Design review of the part built by this model. Coordinates are the model's own, in mm. Give positions to 0.01 mm unless a question says otherwise; leave off trailing zeros. Write each loop counter-clockwise with the first axis right and the second up, starting at its lowest first coordinate (ties: lowest second). Pieces come first, ordered by that corner, then holes. Notation, with made-up numbers: M 65.5,35.25 L 116.5,35.25 A15 cw 116.5,48.25 Z; hole C -4.5,1 d2. An arc over 180 degrees is marked long. Write each question's results on one line, items separated by ' | '. Start each with the question number.
from build123d import *

# Parameters (mm, degrees)
F0_W     = 15
F0_H     = 3.175
F0_W_2   = 10
F0_W_3   = 11
F0_H_2   = 20
F1_DEPTH = 3.175
F2_R     = 5


# Not quite as in the source:
# - a feature names something its author has since deleted; it is built from what else it names


with BuildPart() as f1:
    # F0 (on Right) → F1 (new body)
    with BuildSketch(Plane.YZ):
        with Locations((-94.0358207209, -1.5875)):
            Rectangle(F0_W, F0_H)
        with Locations((-64.0358207209, -1.5875)):
            Rectangle(F0_W, F0_H)
        with Locations((-34.0358207209, -1.5875)):
            Rectangle(F0_W, F0_H)
        with Locations((-4.0358207209, -1.5875)):
            Rectangle(F0_W, F0_H)
        Polygon((-101.5358207209, 20), (-101.5358207209, 0), (-86.5358207209, 0), (-71.5358207209, 0), (-56.5358207209, 0), (-41.5358207209, 0), (-26.5358207209, 0), (-11.5358207209, 0), (3.4641792791, 0), (21.4992204921, 0), (38.0393435029, 0), (73.4641792791, 0), (108.4641792791, 0), (108.4641792791, 20), (93.4641792791, 20), (78.4641792791, 20), (63.4641792791, 20), (48.4641792791, 20), (33.4641792791, 20), (18.4641792791, 20), (3.4641792791, 20), (-11.5358207209, 20), (-26.5358207209, 20), (-41.5358207209, 20), (-56.5358207209, 20), (-71.5358207209, 20), (-86.5358207209, 20), align=None)
        with Locations((29.5455027372, 3.4310361944)):
            Rectangle(F0_W_2, F0_H, mode=Mode.SUBTRACT)
        with Locations((59.5455027372, 3.4310361944)):
            Rectangle(F0_W_2, F0_H, mode=Mode.SUBTRACT)
        with Locations((89.5455027372, 3.4310361944)):
            Rectangle(F0_W_2, F0_H, mode=Mode.SUBTRACT)
        Polygon((38.0393435029, 0), (21.4992204921, 0), (21.4992204921, -50), (73.4641792791, -50), (73.4641792791, -35), (73.4641792791, 0), align=None)
        with Locations((30.0455027372, -34.3287487835)):
            Rectangle(F0_W_3, F0_H, mode=Mode.SUBTRACT)
        with Locations((60.0455027372, -34.3287487835)):
            Rectangle(F0_W_3, F0_H, mode=Mode.SUBTRACT)
        with Locations((29.5455027372, -14.3287487835)):
            Rectangle(F0_W_2, F0_H, mode=Mode.SUBTRACT)
        with Locations((59.5455027372, -14.3287487835)):
            Rectangle(F0_W_2, F0_H, mode=Mode.SUBTRACT)
        with Locations((-94.0358207209, 21.5875)):
            Rectangle(F0_W, F0_H)
        with Locations((-64.0358207209, 21.5875)):
            Rectangle(F0_W, F0_H)
        with Locations((-34.0358207209, 21.5875)):
            Rectangle(F0_W, F0_H)
        with Locations((-4.0358207209, 21.5875)):
            Rectangle(F0_W, F0_H)
        with Locations((25.9641792791, 21.5875)):
            Rectangle(F0_W, F0_H)
        with Locations((55.9641792791, 21.5875)):
            Rectangle(F0_W, F0_H)
        with Locations((85.9641792791, 21.5875)):
            Rectangle(F0_W, F0_H)
        with Locations((115.9641792791, 21.5875)):
            Rectangle(F0_W, F0_H)
        with Locations((115.9641792791, 10)):
            Rectangle(F0_W, F0_H_2)
        Polygon((73.4641792791, -35), (73.4641792791, -50), (123.4641792791, 0), (108.4641792791, 0), align=None)
    extrude(amount=F1_DEPTH)

    # F2
    f2_edges = [f1.edges().sort_by_distance(p)[0] for p in [
        (1.5875, 123.464179, 0),
        (1.5875, 73.464179, -50),
        (1.5875, 21.49922, -50),
    ]]
    fillet(f2_edges, radius=F2_R)


solid = f1.part
Q1. We need section A-A on y = 90.5. Write out the cut boundary in (x, z) (3 decimals), and give its area (3 significant figures).
Q2. For pin 1 Ø1.6 at (x, y) = (1, -79.5) entering from -Z; pin 2 Ø1 at (x, y) = (1.5, -95.5) entering from -Z (3 decimals); pin 3 Ø1.5 at (x, z) = (2.5, -29.5) entering from -Y, all flat-tipped, find the tip position at first contact; note any pin that passes through.
Q3. We need section D-D on y = -7. Write out the cut boundary in (x, z) (3 decimals).
Q4. We need section C-C on x = 1.25. Count the separate pieces of the cut face and the enclosed holes in it, and give its area (3 significant figures).
Q5. The part is to be moulded in two halves that separate along Y. For faces 1 (the flat face through (1.565, 98.135, -25.329)), 2 (the cylindrical face through (1.61, 22.93, -48.5)), 3 (the flat face through (1.565, 91.209, -17.255)), say which applies: pulls with the +Y half, pulls with the -Y half, needs draft (parallel to the pull), parting line crosses it, or undercut.
Q6. Wall thickness on line 1 along Z through (x, y) = (0.2, 57.5) (3 decimals); line 2 along Y through (x, z) = (3, -15); line 3 along Y through (x, z) = (2.4, -33.5): over which ranges is each line inside the solid? List them lowest first. Write a range as from..to.
Q7. We need section B-B on z = -24. Write out the cut boundary in (x, y) (3 decimals).
Answer sheet:
1) outline: M 0,-32.964 L 3.175,-32.964 L 3.175,-17.964 L 0,-17.964 Z; M 0,0 L 3.175,0 L 3.175,1.844 L 0,1.844 Z; M 0,5.019 L 3.175,5.019 L 3.175,23.175 L 0,23.175 Z | area: 111 mm^2
2) pin 1: z = 0 | pin 2: z = -3.175 | pin 3: y = 21.5
3) outline: M 0,-3.175 L 3.175,-3.175 L 3.175,23.175 L 0,23.175 Z
4) separate pieces: 1 | enclosed holes: 8 | area: 8,070 mm^2
5) face 1: pulls with the +Y half | face 2: pulls with the -Y half | face 3: undercut
6) line 1: -50..-35.916, -32.741..-15.916, -12.741..1.844, 5.019..23.175 | line 2: 21.5..24.55, 34.55..54.55, 64.55..73.46, 93.46..108.46 | line 3: 21.5..24.55, 35.55..54.55, 65.55..73.46, 74.96..89.96
7) outline: M 0,21.499 L 3.175,21.499 L 3.175,73.464 L 0,73.464 Z; M 0,84.464 L 3.175,84.464 L 3.175,99.464 L 0,99.464 Z
